from build123d import *

# Parameters (mm, degrees)
SKETCH1_R                = 1
BOSS_EXTRUDE1_DEPTH      = 4
BOSS_EXTRUDE2_DEPTH      = 1.5
BOSS_EXTRUDE2_DEPTH_BACK = 1.5
BOSS_EXTRUDE2_START      = 2
SKETCH2_R                = 1
SKETCH3_W                = 1
SKETCH3_H                = 6.076691854
CUT_EXTRUDE1_DEPTH       = 10


with BuildPart() as part:
    # Sketch1 → Boss-Extrude1 (new body)
    with BuildSketch(Plane.XY):
        with BuildLine():
            Line((-2.5, 0), (-2.5, 3.5))
            ThreePointArc((-2.5, 3.5), (-2.060660172, 4.560660172), (-1, 5))
            Line((-1, 5), (1, 5))
            ThreePointArc((1, 5), (2.060660172, 4.560660172), (2.5, 3.5))
            Line((2.5, 3.5), (2.5, 0))
            ThreePointArc((2.5, 0), (0, -2.5), (-2.5, 0))
        make_face()
        Circle(SKETCH1_R, mode=Mode.SUBTRACT)
    extrude(amount=BOSS_EXTRUDE1_DEPTH)

    # Sketch2 → Boss-Extrude2 (add, two sides: drawn at the far end of the back side and taken through both)
    with BuildSketch(Plane.XY.offset(BOSS_EXTRUDE2_START - BOSS_EXTRUDE2_DEPTH_BACK)):
        with BuildLine():
            Line((1, 5), (1, 20))
            ThreePointArc((1, 20), (1.192761143, 26.644591422), (-2.91696209, 21.419849613))
            Line((-2.91696209, 21.419849613), (-1, 18.528962219))
            Line((-1, 18.528962219), (-1, 5))
            Line((-1, 5), (1, 5))
        make_face()
        with Locations((0, 23.354101966)):
            Circle(SKETCH2_R, mode=Mode.SUBTRACT)
    extrude(amount=BOSS_EXTRUDE2_DEPTH + BOSS_EXTRUDE2_DEPTH_BACK)

    # Sketch3 → Cut-Extrude1 (cut)
    with BuildSketch(Plane(origin=(2.5, 0, 0), x_dir=(0, 0, -1), z_dir=(1, 0, 0))):
        with Locations((-2, -0.507860796)):
            Rectangle(SKETCH3_W, SKETCH3_H)
    extrude(amount=-CUT_EXTRUDE1_DEPTH, mode=Mode.SUBTRACT)


solid = part.part
Could you check a few things on this model? Use its own coordinates, in mm. A direction names the side the tool comes from. Round coordinates to 2 decimals unless told otherwise and drop trailing zeros. Write each loop counter-clockwise with the first axis right and the second up, starting at its lowest first coordinate (ties: lowest second). Pieces come first, ordered by that corner, then holes. Notation, with made-up numbers: (-26.5, 68.25) -> (-9.5, 68.25) arc R8 ccw to (-9.5, 83.25) -> close; hole circle Ø9 at (33.5, -7). An arc over 180 degrees is marked (long way). Use a Markdown table: item, result.
1. If we section it at A-A (x = 0): List the corners of the cut face in (y, z) for me.
Answer key:
| item | result |
|---|---|
| outline | (-2.5, 0) -> (-1, 0) -> (-1, 1.5) -> (-2.5, 1.5) -> close; (-2.5, 2.5) -> (-1, 2.5) -> (-1, 4) -> (-2.5, 4) -> close; (1, 0) -> (5, 0) -> (5, 0.5) -> (22.35, 0.5) -> (22.35, 3.5) -> (5, 3.5) -> (5, 4) -> (1, 4) -> (1, 2.5) -> (2.53, 2.5) -> (2.53, 1.5) -> (1, 1.5) -> close; (24.35, 0.5) -> (26.85, 0.5) -> (26.85, 3.5) -> (24.35, 3.5) -> close |
2. Which directions (+Z, -Z, +X, -X, +Y, -Y) give clear straight access to the entire face, cutting with the end or side of a thin tool? Please do faces 1 (the face through (0, 19, 3.5)), 2 (the face through (2.05, 4.57, 1.97)), 3 (the face through (-1.97, 19.99, 1.98)).
Answer key:
| item | result |
|---|---|
| face 1 | +Z, +X, -X, +Y |
| face 2 | +Z, -Z, +X |
| face 3 | +Z, -Z, -X |
3. If we section it at C-C (z = 3.25): List the corners of the cut face in (x, y) for me.
Answer key:
| item | result |
|---|---|
| outline | (-2.92, 21.42) -> (-1, 18.53) -> (-1, 5) arc R1.5 ccw to (-2.5, 3.5) -> (-2.5, 0) arc R2.5 ccw to (2.5, 0) -> (2.5, 3.5) arc R1.5 ccw to (1, 5) -> (1, 20) arc R3.5 ccw (long way) to start; hole circle Ø2 at (0, 0); hole circle Ø2 at (0, 23.35) |
4. Please list where these lines run through material, in increasing order: probe 1 along Y at (x, z) = (0, 3.25); probe 2 along X at (y, z) = (0, 3.4); probe 3 along Z at (x, y) = (0.25, 17.75).
Answer key:
| item | result |
|---|---|
| probe 1 | y = -2.5 to -1, 1 to 22.35, 24.35 to 26.85 |
| probe 2 | x = -2.5 to -1, 1 to 2.5 |
| probe 3 | z = 0.5 to 3.5 |
5. If we section it at D-D (y = 10.25): List the corners of the cut face in (x, z) for me.
Answer key:
| item | result |
|---|---|
| outline | (-1, 0.5) -> (1, 0.5) -> (1, 3.5) -> (-1, 3.5) -> close |
6. If we section it at B-B (x = -1.75): List the corners of the cut face in (y, z) for me, then the cut area to 3 significant figures.
Answer key:
| item | result |
|---|---|
| outline | (-1.79, 0) -> (4.8, 0) -> (4.8, 4) -> (-1.79, 4) -> (-1.79, 2.5) -> (2.53, 2.5) -> (2.53, 1.5) -> (-1.79, 1.5) -> close; (19.66, 0.5) -> (26.39, 0.5) -> (26.39, 3.5) -> (19.66, 3.5) -> close |
| area | 42.2 mm^2 |
7. For pin 1 Ø2 at (y, z) = (12, 3.5) entering from +X; pin 2 Ø1.1 at (x, z) = (-0.5, 2) entering from -Y; pin 3 Ø1.2 at (x, y) = (0, 0) entering from -Z; pin 4 Ø1 at (y, z) = (1, 2.5) entering from +X, each with a flat end and sliding along its axis, tell me the tip position at first contact or that it passes through.
Answer key:
| item | result |
|---|---|
| pin 1 | stops at x = 1 |
| pin 2 | stops at y = -2.49 |
| pin 3 | passes through |
| pin 4 | stops at x = 2.5 |
8. We'd pull the mould along X, two halves only. Please class faces 4 (the face through (0, -1, 1)), 5 (the face through (2.5, 3, 2)), 6 (the face through (-1, 1, 1.5)), 7 (the face through (0, -1, 3)): +X half, -X half, draft (parallel to the pull), parting line (faces both ways), or undercut.
Answer key:
| item | result |
|---|---|
| face 4 | undercut |
| face 5 | +X half |
| face 6 | draft |
| face 7 | undercut |
